Build history of the part. All positions in model axes, mm. A direction names the side the tool comes from. Give positions to 0.01 mm unless a question says otherwise; leave off trailing zeros. Order: outer loops, then holes, each group sorted by start corner. A loop starts at its lowest first (then second) coordinate and runs counter-clockwise, first axis right, second up. Notation, with made-up numbers: (-10.5, -1.75) - (12.5, -1.75) arc R23 ccw to (12.5, 34.25) - close; hole circle Ø1 at (37.5, -34). An arc over 180 degrees is marked (long way). Answer in a Markdown table with one row per item.
```python
from build123d import *

# Parameters (mm, degrees)
F0_W     = 55
F0_H     = 55
F1_DEPTH = 7
F4_DEPTH = 10
F3_R     = 2
F5_DEPTH = 7.001


with BuildPart() as f1:
    # F0 (on Top) → F1 (new body)
    with BuildSketch(Plane.XY):
        with Locations((-27.5, 27.5)):
            Rectangle(F0_W, F0_H)
    extrude(amount=F1_DEPTH)

    # F2 (on face) → F4 (join)
    with BuildSketch(Plane.XY.offset(7)):
        with BuildLine():
            Line((-43.1786440313, 18.3423049748), (-43.1786440313, 36.1469540578))
            ThreePointArc((-43.1786440313, 36.1469540578), (-47.3423168357, 41.6235479841), (-48.8213559687, 48.3423049748))
            Line((-48.8213559687, 48.3423049748), (-53.8213559687, 48.3423049748))
            Line((-53.8213559687, 48.3423049748), (-53.8213559687, 18.3423049748))
            Line((-53.8213559687, 18.3423049748), (-43.1786440313, 18.3423049748))
        make_face()
        with BuildLine():
            Line((-27.5, 18.3423049748), (-27.5, 33.2531310195))
            ThreePointArc((-27.5, 33.2531310195), (-35.7254403266, 32.6080654303), (-43.1786440313, 36.1469540578))
            Line((-43.1786440313, 36.1469540578), (-43.1786440313, 18.3423049748))
            Line((-43.1786440313, 18.3423049748), (-27.5, 18.3423049748))
        make_face()
        with BuildLine():
            ThreePointArc((-16.8213559687, 48.3423049748), (-19.7610784927, 39.0995157718), (-27.5, 33.2531310195))
            ThreePointArc((-27.5, 33.2531310195), (-19.2745596734, 32.6080654303), (-11.8213559687, 36.1469540578))
            Line((-11.8213559687, 36.1469540578), (-11.8213559687, 48.3423049748))
            Line((-11.8213559687, 48.3423049748), (-16.8213559687, 48.3423049748))
        make_face()
        with BuildLine():
            ThreePointArc((-11.8213559687, 36.1469540578), (-19.2745596734, 32.6080654303), (-27.5, 33.2531310195))
            Line((-27.5, 33.2531310195), (-27.5, 18.3423049748))
            Line((-27.5, 18.3423049748), (-11.8213559687, 18.3423049748))
            Line((-11.8213559687, 18.3423049748), (-11.8213559687, 36.1469540578))
        make_face()
    extrude(amount=F4_DEPTH)

    # F3 (on face) → F5 (cut, through all)
    with BuildSketch(Plane.XY.offset(7)):
        with Locations((-20.5813342872, 9.34450762)):
            Circle(F3_R)
        with Locations((-5.5655137111, 9.34450762)):
            Circle(F3_R)
        with Locations((-5.5655137111, 29.042776674)):
            Circle(F3_R)
        with Locations((-5.5655137111, 45.6509888542)):
            Circle(F3_R)
    extrude(amount=-F5_DEPTH, mode=Mode.SUBTRACT)


solid = f1.part
```
1. Cut at A-A on y = 20.5. Write the cut outline in (x, z), and give its area (3 significant figures).
Check result:
| item | result |
|---|---|
| outline | (-55, 0) - (0, 0) - (0, 7) - (-11.82, 7) - (-11.82, 17) - (-53.82, 17) - (-53.82, 7) - (-55, 7) - close |
| area | 805 mm² |
2. Cut at D-D on x = -20.5. Write the cut outline in (y, z), and give its area (3 significant figures).
Check result:
| item | result |
|---|---|
| outline | (0, 0) - (7.35, 0) - (7.35, 7) - (0, 7) - close; (11.34, 0) - (55, 0) - (55, 7) - (38.14, 7) - (38.14, 17) - (18.34, 17) - (18.34, 7) - (11.34, 7) - close |
| area | 555 mm² |
3. Probe line 1 (X direction, y = 48, z = 12); line 2 (Z direction, x = -31.5, y = 16); line 3 (X direction, y = 23, z = 9.5). List the from-to ranges inside material, lowest first.
Check result:
| item | result |
|---|---|
| line 1 | x = -53.82 to -48.82, -16.83 to -11.82 |
| line 2 | z = 0 to 7 |
| line 3 | x = -53.82 to -11.82 |
4. Cut at B-B on z = 7.75. Write the cut outline in (x, y), and give its area (3 significant figures).
Check result:
| item | result |
|---|---|
| outline | (-53.82, 18.34) - (-11.82, 18.34) - (-11.82, 48.34) - (-16.82, 48.34) arc R16 cw to (-48.82, 48.34) - (-53.82, 48.34) - close |
| area | 858 mm² |
5. Which spindle directions (+Z, -Z, +X, -X, +Y, -Y) get a long thin tool onto all of the face, cutting with end or side? Do faces 4 (the face through (-33, 18.342, 12)), 5 (the face through (-53.821, 34, 12)), 6 (the face through (-5.826, 11.327, 3.549)), 7 (the face through (-14, 48.342, 12)). Say none if no direction does.
Check result:
| item | result |
|---|---|
| face 4 | +Z, +X, -X, -Y |
| face 5 | +Z, -X, +Y, -Y |
| face 6 | +Z, -Z |
| face 7 | +Z, +X, -X, +Y |
6. Cut at C-C on z = 4.75. Write the cut outline in (x, y).
Check result:
| item | result |
|---|---|
| outline | (-55, 0) - (0, 0) - (0, 55) - (-55, 55) - close; hole circle Ø4 at (-20.58, 9.34); hole circle Ø4 at (-5.57, 9.34); hole circle Ø4 at (-5.57, 29.04); hole circle Ø4 at (-5.57, 45.65) |
7. Two-plate mould, pull along X, no slides. Class faces 1 (the face through (-11.821, 33, 12)), 2 (the face through (-18.674, 9.945, 3.549)), 3 (the face through (-28, 28, 0)): +X half, -X half, draft (parallel to the pull), parting line (faces both ways), or undercut.
Check result:
| item | result |
|---|---|
| face 1 | +X half |
| face 2 | undercut |
| face 3 | draft |
8. Drop flat-ended pins along their axis: P1, Ø1.5, axis at x = -36, z = 8.5, coming from the +Y side; P2, Ø4, axis at x = -52, z = 13.5, coming from the +Y side; P3, Ø3, axis at x = -34, z = 14, coming from the -Y side; P4, Ø3, axis at x = -5.57, y = 9.34, coming from the -Z side. Give the stop position or say it passes through.
Check result:
| item | result |
|---|---|
| P1 | stops at y = 32.83 |
| P2 | stops at y = 48.34 |
| P3 | stops at y = 18.34 |
| P4 | passes through |
